```python
from build123d import *

# Parameters (mm, degrees)
SKIZZE1_W                       = 300
SKIZZE1_H                       = 150
AUFSATZ_LINEAR_AUSTRAGEN1_DEPTH = 5
SKIZZE2_R                       = 1.5
SKIZZE2_W                       = 28
SKIZZE2_H                       = 20
SCHNITT_LINEAR_AUSTRAGEN1_DEPTH = 168.779617356
SKIZZE3_R                       = 11
SCHNITT_LINEAR_AUSTRAGEN2_DEPTH = 168.779617356
SKIZZE4_R                       = 1
SCHNITT_LINEAR_AUSTRAGEN3_DEPTH = 168.779617356
SKIZZE5_R                       = 2.5
SKIZZE5_W                       = 55
SKIZZE5_H                       = 46
SCHNITT_LINEAR_AUSTRAGEN4_DEPTH = 168.779617356
SKIZZE6_R                       = 1
SCHNITT_LINEAR_AUSTRAGEN5_DEPTH = 168.779617356
SCHNITT_LINEAR_AUSTRAGEN6_DEPTH = 168.779617356
FASE1_SIZE                      = 2.5


with BuildPart() as part:
    # Skizze1 → Aufsatz-Linear austragen1 (new body)
    with BuildSketch(Plane.XY):
        Rectangle(SKIZZE1_W, SKIZZE1_H)
    extrude(amount=AUFSATZ_LINEAR_AUSTRAGEN1_DEPTH)

    # Skizze2 → Schnitt-Linear austragen1 (cut, through all)
    with BuildSketch(Plane.XY.offset(5)):
        with Locations((-121, -50)):
            Circle(SKIZZE2_R)
        with Locations((-81, -50)):
            Circle(SKIZZE2_R)
        with Locations((-101, -50)):
            Rectangle(SKIZZE2_W, SKIZZE2_H)
    extrude(amount=-SCHNITT_LINEAR_AUSTRAGEN1_DEPTH, mode=Mode.SUBTRACT)

    # Skizze3 → Schnitt-Linear austragen2 (cut, through all)
    with BuildSketch(Plane.XY.offset(5)):
        with Locations((110, -45)):
            Circle(SKIZZE3_R)
        with Locations((70, -45)):
            Circle(SKIZZE3_R)
    extrude(amount=-SCHNITT_LINEAR_AUSTRAGEN2_DEPTH, mode=Mode.SUBTRACT)

    # Skizze4 → Schnitt-Linear austragen3 (cut, through all)
    with BuildSketch(Plane.XY.offset(5)):
        with Locations((-115, -40)):
            Circle(SKIZZE4_R)
        with Locations((-87, -40)):
            Circle(SKIZZE4_R)
        with Locations((-87, -60)):
            Circle(SKIZZE4_R)
        with Locations((-115, -60)):
            Circle(SKIZZE4_R)
    extrude(amount=-SCHNITT_LINEAR_AUSTRAGEN3_DEPTH, mode=Mode.SUBTRACT)

    # Skizze5 → Schnitt-Linear austragen4 (cut, through all)
    with BuildSketch(Plane.XY.offset(5)):
        with Locations((-61, -17)):
            Circle(SKIZZE5_R)
        with Locations((14, -17)):
            Circle(SKIZZE5_R)
        with Locations((-23.5, -17)):
            Rectangle(SKIZZE5_W, SKIZZE5_H)
    extrude(amount=-SCHNITT_LINEAR_AUSTRAGEN4_DEPTH, mode=Mode.SUBTRACT)

    # Skizze6 → Schnitt-Linear austragen5 (cut, through all)
    with BuildSketch(Plane.XY.offset(5)):
        with Locations((-51, 6)):
            Circle(SKIZZE6_R)
        with Locations((4, 6)):
            Circle(SKIZZE6_R)
        with Locations((4, -40)):
            Circle(SKIZZE6_R)
        with Locations((-51, -40)):
            Circle(SKIZZE6_R)
    extrude(amount=-SCHNITT_LINEAR_AUSTRAGEN5_DEPTH, mode=Mode.SUBTRACT)

    # Skizze7 → Schnitt-Linear austragen6 (cut, through all)
    with BuildSketch(Plane.XY.offset(5)):
        with BuildLine():
            Line((30, -40.645898034), (29, -41.645898034))
            ThreePointArc((29, -41.645898034), (30, -48.5), (31, -41.645898034))
            Line((31, -41.645898034), (30, -40.645898034))
        make_face()
    extrude(amount=-SCHNITT_LINEAR_AUSTRAGEN6_DEPTH, mode=Mode.SUBTRACT)

    # Fase1
    fase1_edges = [part.edges().sort_by_distance(p)[0] for p in [
        (-63.5, -17, 0),
        (11.5, -17, 0),
    ]]
    chamfer(fase1_edges, length=FASE1_SIZE)


solid = part.part
```
Input: part model. Units: mm. Frame: model coordinates. Coordinates: 2 decimals unless noted, no trailing zeros. Loops run counter-clockwise (first coordinate to the right, second up) from the corner with the lowest first, then second, coordinate; pieces in that order, holes last. Notation, with made-up numbers: (89.25, 1) - (128.25, 1) arc R23 cw to (128.25, 33) - close; hole circle Ø9 at (0, -8.75). An arc over 180 degrees is marked (long way). Answer in a Markdown table with one row per item.
(1) Material intervals for L1, parallel to X at y = -38, z = 3.3; L2, parallel to Y at x = 110, z = 1.5; L3, parallel to Y at x = -101.5, z = 2.85, sorted ascending. Write a range as from..to.
Model answer:
| item | result |
|---|---|
| L1 | x = -150..-51, 4..61.51, 78.49..101.51, 118.49..150 |
| L2 | y = -75..-56, -34..75 |
| L3 | y = -75..-60, -40..75 |
(2) Cut plane B-B on z = 1.25. Count the separate pieces of the cut face and the enclosed holes in it, plus the area to 3 significant figures.
Model answer:
| item | result |
|---|---|
| separate pieces | 1 |
| enclosed holes | 9 |
| area | 41,000 mm² |
(3) Pin query (flat end, axial travel): P1, Ø1.8, axis at x = -115, y = -40, coming from the +Z side; P2, Ø2.5, axis at x = -51, y = -40, coming from the +Z side. Return the tip coordinate at first contact, or that it passes through.
Model answer:
| item | result |
|---|---|
| P1 | passes through |
| P2 | stops at z = 5 |
(4) Mould query, pull axis X, two halves, no side actions, for faces 1 (the face through (-2, 18, 5)), 2 (the face through (59, -45, 3)). Classes: pulls with the +X half, pulls with the -X half, needs draft (parallel to the pull), parting line crosses it, or undercut.
Model answer:
| item | result |
|---|---|
| face 1 | needs draft |
| face 2 | undercut |
(5) Cut plane A-A on y = -45. Output: boundary loops of the cut face in (x, z), plus the area to 4 significant figures.
Model answer:
| item | result |
|---|---|
| outline | (-150, 0) - (-115, 0) - (-115, 5) - (-150, 5) - close; (-87, 0) - (26.5, 0) - (26.5, 5) - (-87, 5) - close; (33.5, 0) - (59, 0) - (59, 5) - (33.5, 5) - close; (81, 0) - (99, 0) - (99, 5) - (81, 5) - close; (121, 0) - (150, 0) - (150, 5) - (121, 5) - close |
| area | 1,105 mm² |
